from build123d import *

# Parameters (mm, degrees)
F0_W     = 127
F0_H     = 127
F1_DEPTH = 63.5
F2_DEPTH = 63.5
F3_R     = 12.7
F4_R     = 12.7
F5_DEPTH = 127
F6_R     = 12.7
F7_DEPTH = 127
F8_R     = 12.7
F9_DEPTH = 381


with BuildPart() as f1:
    # F0 (on Top) → F1 (new body)
    with BuildSketch(Plane.XY):
        Rectangle(F0_W, F0_H)
    extrude(amount=F1_DEPTH)

    # F2 (add): faces of the model
    f2_faces = [f1.faces().sort_by_distance(p)[0] for p in [
        (0, 0, 0),
        (0, 0, 63.5),
    ]]
    extrude(f2_faces, amount=F2_DEPTH, dir=(0, 0, -1))

    # F3
    f3_edges = [f1.edges().sort_by_distance(p)[0] for p in [
        (0, -63.5, 63.5),
        (-63.5, 0, 63.5),
        (-63.5, -63.5, 0),
        (0, 63.5, 63.5),
        (63.5, 0, 63.5),
        (63.5, 63.5, 0),
        (63.5, -63.5, 0),
        (63.5, 0, -63.5),
        (0, -63.5, -63.5),
        (-63.5, 63.5, 0),
        (0, 63.5, -63.5),
        (-63.5, 0, -63.5),
    ]]
    fillet(f3_edges, radius=F3_R)

    # F4 (on face) → F5 (cut)
    with BuildSketch(Plane.XY.offset(63.5)):
        Circle(F4_R)
    extrude(amount=-F5_DEPTH, mode=Mode.SUBTRACT)

    # F6 (on face) → F7 (cut)
    with BuildSketch(Plane.XZ.offset(63.5)):
        Circle(F6_R)
    extrude(amount=-F7_DEPTH, mode=Mode.SUBTRACT)

    # F8 (on face) → F9 (cut)
    with BuildSketch(Plane.YZ.offset(63.5)):
        Circle(F8_R)
    extrude(amount=-F9_DEPTH, mode=Mode.SUBTRACT)


solid = f1.part
Geometry: final body of the model. Coordinates: model frame, mm. Give positions to 0.01 mm unless a question says otherwise; leave off trailing zeros. Loops run counter-clockwise (first coordinate to the right, second up) from the corner with the lowest first, then second, coordinate; pieces in that order, holes last. Notation, with made-up numbers: (72.25, -27.75) - (103.25, -27.75) arc R25 cw to (103.25, -13.75) - close; hole circle Ø3 at (7, 8.5). An arc over 180 degrees is marked (long way). Answer as CSV lines item,"result". Start each with the question number.
1. Section C-C, the plane z = 39.5. Return loops of the section in (x, y), plus the area to 3 significant figures.
2. Section A-A, the plane y = 0. Return loops of the section in (x, z).
3. Draft query along X for faces 1 (the face through (0.71, 59.68, 59.88)), 2 (the face through (12.114, 3.815, 36.622)), 3 (the face through (59.88, 59.68, -0.71)). Return one class per face: released by +X, released by -X, zero draft, split by the parting line, or undercut.
4. Ray query, L1, parallel to X at y = 0, z = -40.5. Return the intervals inside material, ascending.
5. Pin query (flat end, axial travel): P1, Ø23, axis at x = 0, z = 0, coming from the +Y side. Return the tip coordinate at first contact, or that it passes through.
Answers:
1,outline,"(-63.5, -50.8) arc R12.7 ccw to (-50.8, -63.5) - (50.8, -63.5) arc R12.7 ccw to (63.5, -50.8) - (63.5, 50.8) arc R12.7 ccw to (50.8, 63.5) - (-50.8, 63.5) arc R12.7 ccw to (-63.5, 50.8) - close; hole circle Ø25.4 at (0, 0)"
1,area,"15,500 mm2"
2,outline,"(-63.5, -50.8) arc R12.7 ccw to (-50.8, -63.5) - (-12.7, -63.5) - (-12.7, -12.7) - (-63.5, -12.7) - close; (-63.5, 12.7) - (-12.7, 12.7) - (-12.7, 63.5) - (-50.8, 63.5) arc R12.7 ccw to (-63.5, 50.8) - close; (12.7, -63.5) - (50.8, -63.5) arc R12.7 ccw to (63.5, -50.8) - (63.5, -12.7) - (12.7, -12.7) - close; (12.7, 12.7) - (63.5, 12.7) - (63.5, 50.8) arc R12.7 ccw to (50.8, 63.5) - (12.7, 63.5) - close"
3,face 1,"zero draft"
3,face 2,"undercut"
3,face 3,"released by +X"
4,L1,"x = -63.5 to -12.7, 12.7 to 63.5"
5,P1,"passes through"
